Answer from the drawing. Dimensions are ordinates in mm from the lowest x, y and z of the part. Round coordinates to 2 decimals unless told otherwise and drop trailing zeros. Write each loop counter-clockwise with the first axis right and the second up, starting at its lowest first coordinate (ties: lowest second). Pieces come first, ordered by that corner, then holes. Notation, with made-up numbers: (13, 86) - (64, 86) arc R30 cw to (64, 108) - close; hole circle Ø8 at (27, 80). An arc over 180 degrees is marked (long way). One line per item, written item: value. Start each with the question number.
(1) A cutting plane is placed at C-C, the plane y = 36. Determine the outline of the cut face in (x, z), plus the area to 3 significant figures.
(2) Flat-ended cylindrical pins translate along their axes: pin 1 Ø1.3 at (y, z) = (9, 2) entering from +X; pin 2 Ø2 at (x, z) = (52.5, 3) entering from -Y; pin 3 Ø2 at (x, z) = (52.5, 1.5) entering from +Y. Find the tip coordinate at first contact, or state that the pin passes through.
(3) A cutting plane is placed at A-A, the plane x = 20. Determine the outline of the cut face in (y, z) (1 decimal).
(4) A cutting plane is placed at B-B, the plane z = 1.7. Determine the outline of the cut face in (x, y) (1 decimal).
(5) A cutting plane is placed at D-D, the plane x = 10.5. Determine the outline of the cut face in (y, z), plus the area to 3 significant figures.
(6) Find the intervals of material crossed by L1, parallel to Y at x = 51, z = 1.25; L2, parallel to Y at x = 20, z = 3.05 (1 decimal); L3, parallel to X at y = 17, z = 3.6 (1 decimal), in increasing order.
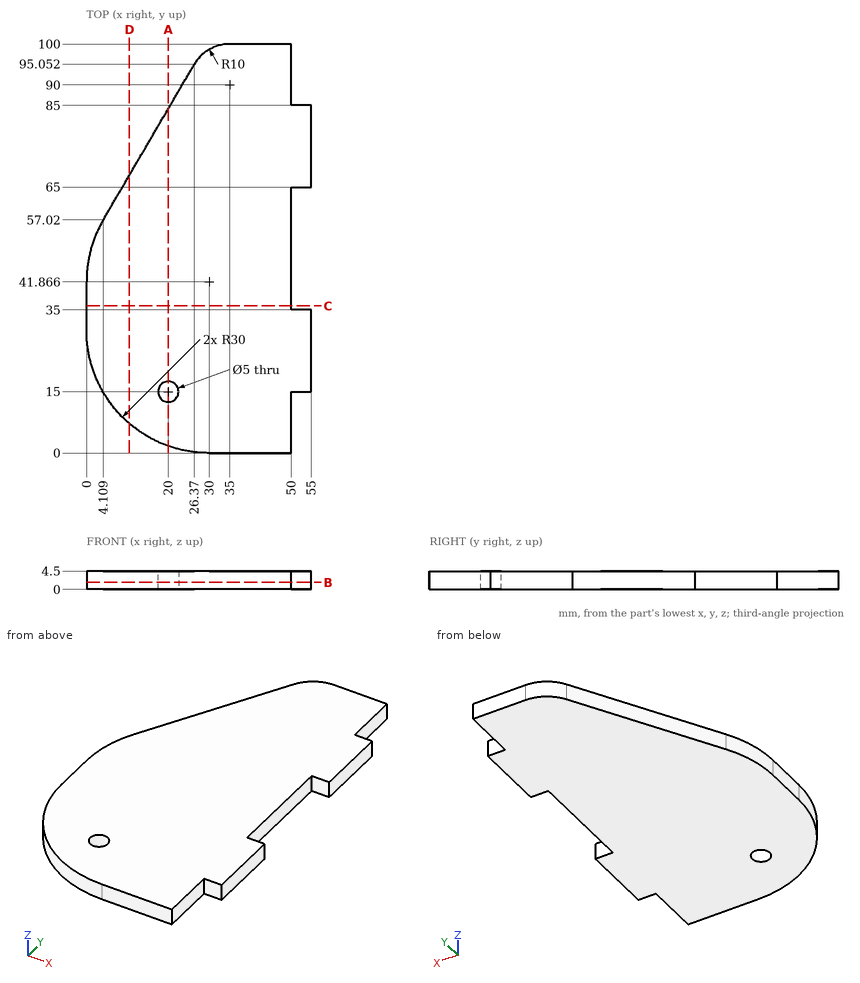
Here are the results:
1. outline: (0, 0) - (50, 0) - (50, 4.5) - (0, 4.5) - close
1. area: 225 mm²
2. pin 1: x = 50
2. pin 2: y = 15
2. pin 3: y = 85
3. outline: (1.7, 0) - (12.5, 0) - (12.5, 4.5) - (1.7, 4.5) - close; (17.5, 0) - (84.2, 0) - (84.2, 4.5) - (17.5, 4.5) - close
4. outline: (0, 30) arc R30 ccw to (30, 0) - (50, 0) - (50, 15) - (55, 15) - (55, 35) - (50, 35) - (50, 65) - (55, 65) - (55, 85) - (50, 85) - (50, 100) - (35, 100) arc R10 ccw to (26.4, 95.1) - (4.1, 57) arc R30 ccw to (0, 41.9) - close; hole circle Ø5 at (20, 15)
5. outline: (7.2, 0) - (67.94, 0) - (67.94, 4.5) - (7.2, 4.5) - close
5. area: 273 mm²
6. L1: 15 to 35, 65 to 85
6. L2: 1.7 to 12.5, 17.5 to 84.2
6. L3: 3 to 18.5, 21.5 to 55
